Input: part model. Units: mm. Frame: model coordinates. Face numbers are marked on the shaded views. A direction names the side the tool comes from. Round coordinates to 2 decimals unless told otherwise and drop trailing zeros. Write each loop counter-clockwise with the first axis right and the second up, starting at its lowest first coordinate (ties: lowest second). Pieces come first, ordered by that corner, then holes. Notation, with made-up numbers: (-35.75, 55.25) -> (21.25, 55.25) arc R16 cw to (21.25, 65.25) -> close; hole circle Ø11 at (57, 73). An arc over 180 degrees is marked (long way). Use CSV: the item, a comma, the result in double quotes.
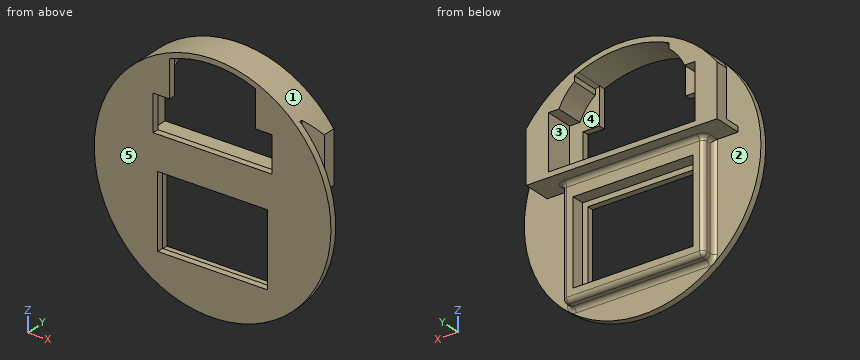
```python
from build123d import *

# Parameters (mm, degrees)
SKETCH1_R               = 27.5
SKETCH1_W               = 25.5
SKETCH1_H               = 17
BOSS_EXTRUDE1_DEPTH     = 1.5
BOSS_EXTRUDE2_START     = 6.6
BOSS_EXTRUDE2_DEPTH     = 6.6
CUT_EXTRUDE1_REACH      = 45.381
CUT_EXTRUDE1_END_RADIUS = 27.5
SKETCH1_5_W             = 32.9
SKETCH1_5_H             = 25.4
SKETCH1_5_W_2           = 27.9
SKETCH1_5_H_2           = 19.4
BOSS_EXTRUDE3_DEPTH     = 3
FILLET1_R               = 1


with BuildPart() as part:
    # Sketch1 → Boss-Extrude1 (new body)
    with BuildSketch(Plane(origin=(0, 0, 0), x_dir=(1, 0, 0), z_dir=(0, 1, 0))):
        with Locations(Location((0, 11.695639977, 0), (0, 0, 270))):
            Circle(SKETCH1_R)
        with BuildLine():
            Line((10, -4.1), (10, -12.629038849))
            ThreePointArc((10, -12.629038849), (0, -14.604360023), (-10, -12.629038849))
            Line((-10, -12.629038849), (-10, -4.1))
            Line((-10, -4.1), (-13.837653888, -4.1))
            Line((-13.837653888, -4.1), (-13.837653888, 4.3))
            Line((-13.837653888, 4.3), (13.837653888, 4.3))
            Line((13.837653888, 4.3), (13.837653888, -4.1))
            Line((13.837653888, -4.1), (10, -4.1))
        make_face(mode=Mode.SUBTRACT)
        with Locations((0, 20.7)):
            Rectangle(SKETCH1_W, SKETCH1_H, mode=Mode.SUBTRACT)
    extrude(amount=-BOSS_EXTRUDE1_DEPTH)

    # Sketch1<3> → Boss-Extrude2 (add)
    with BuildSketch(Plane(origin=(0, 0, 0), x_dir=(1, 0, 0), z_dir=(0, 1, 0)).offset(BOSS_EXTRUDE2_START)):
        with BuildLine():
            Line((-16.45, 7.5), (-22.2, 7.5))
            Line((-22.2, 7.5), (-22.2, -4.534270682))
            ThreePointArc((-22.2, -4.534270682), (0, -15.804360023), (22.2, -4.534270682))
            Line((22.2, -4.534270682), (22.2, 7.5))
            Line((22.2, 7.5), (16.45, 7.5))
            Line((16.45, 7.5), (-16.45, 7.5))
        make_face()
        with BuildLine():
            Line((-17, -6.3), (-17, 6.3))
            Line((-17, 6.3), (17, 6.3))
            Line((17, 6.3), (17, -6.3))
            Line((17, -6.3), (14.582906959, -6.3))
            ThreePointArc((14.582906959, -6.3), (13.072174848, -8.850843183), (11, -10.971032764))
            Line((11, -10.971032764), (11, -12.193478885))
            ThreePointArc((11, -12.193478885), (10.502258239, -12.416443547), (10, -12.629038849))
            ThreePointArc((10, -12.629038849), (0, -14.604360023), (-10, -12.629038849))
            ThreePointArc((-10, -12.629038849), (-10.502258239, -12.416443547), (-11, -12.193478885))
            Line((-11, -12.193478885), (-11, -10.971032764))
            ThreePointArc((-11, -10.971032764), (-13.072174848, -8.850843183), (-14.582906959, -6.3))
            Line((-14.582906959, -6.3), (-17, -6.3))
        make_face(mode=Mode.SUBTRACT)
    extrude(amount=-BOSS_EXTRUDE2_DEPTH)

    # Cut-Extrude1: up to this cylinder (the profile starts inside it)
    cut_extrude1_end = Plane(origin=(0, 1.228571, -11.695639977), z_dir=(0, 1, 0)) * Cylinder(CUT_EXTRUDE1_END_RADIUS, 146.762, mode=Mode.PRIVATE)
    # Sketch2 → Cut-Extrude1 (cut, up to the surface)
    with BuildSketch(Plane.XY.offset(-6.3), mode=Mode.PRIVATE) as cut_extrude1_sk1:
        Polygon((-22.2, 3.6), (-19.2, 0.6), (-19.2, 0), (-22.2, 0), align=None)
    cut_extrude1_tool1 = extrude(cut_extrude1_sk1.sketch, amount=CUT_EXTRUDE1_REACH, mode=Mode.PRIVATE) & cut_extrude1_end
    add(cut_extrude1_tool1.solids().sort_by_distance((-21.057143, 1.228571, -6.3))[0], mode=Mode.SUBTRACT)
    # Sketch2 → Cut-Extrude1 (cut, up to the surface)
    with BuildSketch(Plane.XY.offset(-6.3), mode=Mode.PRIVATE) as cut_extrude1_sk2:
        Polygon((19.2, 0.6), (19.2, 0), (22.2, 0), (22.2, 3.6), align=None)
    cut_extrude1_tool2 = extrude(cut_extrude1_sk2.sketch, amount=CUT_EXTRUDE1_REACH, mode=Mode.PRIVATE) & cut_extrude1_end
    add(cut_extrude1_tool2.solids().sort_by_distance((21.057143, 1.228571, -6.3))[0], mode=Mode.SUBTRACT)

    # Sketch1<5> → Boss-Extrude3 (add)
    with BuildSketch(Plane(origin=(0, 0, 0), x_dir=(1, 0, 0), z_dir=(0, 1, 0))):
        with Locations((0, 20.2)):
            Rectangle(SKETCH1_5_W, SKETCH1_5_H)
        with Locations((0, 20.7)):
            Rectangle(SKETCH1_5_W_2, SKETCH1_5_H_2, mode=Mode.SUBTRACT)
    extrude(amount=BOSS_EXTRUDE3_DEPTH)

    # Fillet1
    fillet1_edges = [part.edges().sort_by_distance(p)[0] for p in [
        (16.45, 3, -20.2),
        (16.45, 1.5, -7.5),
        (0, 3, -32.9),
        (16.45, 1.5, -32.9),
        (-16.45, 0, -20.2),
        (-16.45, 1.5, -32.9),
        (-16.45, 1.5, -7.5),
        (-16.45, 3, -20.2),
        (0, 3, -7.5),
        (16.45, 0, -20.2),
        (0, 0, -32.9),
    ]]
    fillet(fillet1_edges, radius=FILLET1_R)


solid = part.part
```
Item 1: Section query C-C on z = -15. Return the cut outline in (x, y).
Worked answers:
outline,"(-27.3, -1.5) -> (-12.75, -1.5) -> (-12.75, 0) -> (-13.95, 0) -> (-13.95, 3) -> (-15.45, 3) arc R1 ccw to (-16.45, 2) -> (-16.45, 1) arc R1 cw to (-17.45, 0) -> (-27.3, 0) -> close; (12.75, -1.5) -> (27.3, -1.5) -> (27.3, 0) -> (17.45, 0) arc R1 cw to (16.45, 1) -> (16.45, 2) arc R1 ccw to (15.45, 3) -> (13.95, 3) -> (13.95, 0) -> (12.75, 0) -> close"
Item 2: Pull-direction query (X, two-part tool) for the marked faces 1, 2 and 3; classes: +X half, -X half, draft (parallel to the pull), parting line (faces both ways), or undercut.
Worked answers:
face 1,"parting line"
face 2,"draft"
face 3,"undercut"
Item 3: Line query: line 1 (X direction, y = 6.25, z = -5); line 2 (Z direction, x = 12.5, y = -1); line 3 (Z direction, x = 0, y = 0.5). Output: solid intervals per line, ascending.
Worked answers:
line 1,"x = -22.2 to -17, 17 to 22.2"
line 2,"z = -36.19 to -29.2, -12.2 to -4.3, 4.1 to 12.8"
line 3,"z = -33.03 to -30.4, -11 to -6.3, 14.6 to 15.8"
Item 4: Set-up query: the marked faces 4 and 5. Return all of +Z, -Z, +X, -X, +Y, -Y with unobstructed straight access to the full face (end or side cutting, diameter ignored); none if empty.
Worked answers:
face 4,"+Y"
face 5,"+Z, -Z, +X, -X, -Y"
Item 5: Section query B-B on z = 1. Return the cut outline in (x, y), plus the area to 3 significant figures.
Worked answers:
outline,"(-24.39, -1.5) -> (-13.84, -1.5) -> (-13.84, 0) -> (-17, 0) -> (-17, 6.6) -> (-22.2, 6.6) -> (-22.2, 3.6) -> (-19.2, 0.6) -> (-19.2, 0) -> (-24.39, 0) -> close; (13.84, -1.5) -> (24.39, -1.5) -> (24.39, 0) -> (19.2, 0) -> (19.2, 0.6) -> (22.2, 3.6) -> (22.2, 6.6) -> (17, 6.6) -> (17, 0) -> (13.84, 0) -> close"
area,"87.7 mm²"
Item 6: Section query D-D on x = 9. Return the cut outline in (y, z).
Worked answers:
outline,"(-1.5, -37.68) -> (0, -37.68) -> (0, -33.9) arc R1 cw to (1, -32.9) -> (2, -32.9) arc R1 ccw to (3, -31.9) -> (3, -30.4) -> (0, -30.4) -> (0, -29.2) -> (-1.5, -29.2) -> close; (-1.5, -12.2) -> (0, -12.2) -> (0, -11) -> (3, -11) -> (3, -8.5) arc R1 cw to (4, -7.5) -> (6.6, -7.5) -> (6.6, -6.3) -> (0, -6.3) -> (0, -4.3) -> (-1.5, -4.3) -> close; (-1.5, 13.02) -> (6.6, 13.02) -> (6.6, 14.29) -> (-1.5, 14.29) -> close"
Item 7: First-contact query: pin 1 Ø23.5 at (x, z) = (-4.5, -15.5) entering from +Y; pin 2 Ø1 at (y, z) = (0, 3) entering from -X; pin 3 Ø0.8 at (y, z) = (-1, -24) entering from +X; pin 4 Ø2 at (y, z) = (3.5, -2) entering from +X. Flat tips, straight axial feed; report the tip coordinate or a pass-through.
Worked answers:
pin 1,"stops at y = 6.6"
pin 2,"stops at x = -23.55"
pin 3,"stops at x = 24.79"
pin 4,"stops at x = 22.2"
Item 8: Section query A-A on x = -1. Return the cut outline in (y, z).
Worked answers:
outline,"(-1.5, -39.18) -> (0, -39.18) -> (0, -33.9) arc R1 cw to (1, -32.9) -> (2, -32.9) arc R1 ccw to (3, -31.9) -> (3, -30.4) -> (0, -30.4) -> (0, -29.2) -> (-1.5, -29.2) -> close; (-1.5, -12.2) -> (0, -12.2) -> (0, -11) -> (3, -11) -> (3, -8.5) arc R1 cw to (4, -7.5) -> (6.6, -7.5) -> (6.6, -6.3) -> (0, -6.3) -> (0, -4.3) -> (-1.5, -4.3) -> close; (-1.5, 14.59) -> (6.6, 14.59) -> (6.6, 15.79) -> (-1.5, 15.79) -> close"
